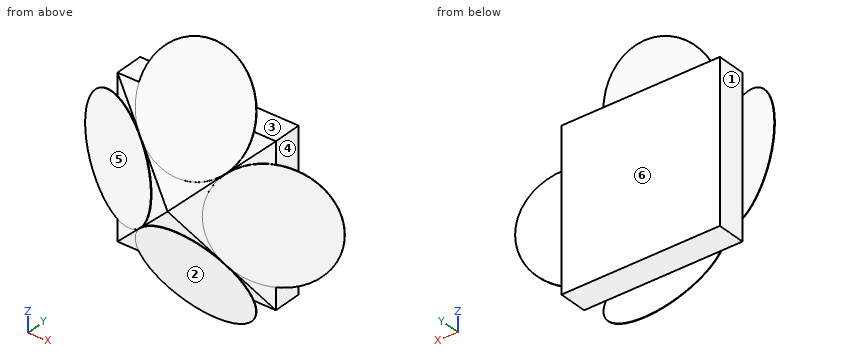
```python
from build123d import *

# Parameters (mm, degrees)
SALIENTE_EXTRUIR1_DEPTH = 32
CORTAR_EXTRUIR1_DEPTH   = 33
CROQUIS3_R              = 11.604472628
SALIENTE_EXTRUIR2_DEPTH = 0.1
CROQUIS4_R              = 11.609993134
SALIENTE_EXTRUIR3_DEPTH = 0.1
CROQUIS6_R              = 11.602426911
SALIENTE_EXTRUIR4_DEPTH = 0.1
CROQUIS7_R              = 11.59621687
SALIENTE_EXTRUIR5_DEPTH = 0.1


with BuildPart() as part:
    # Croquis1 → Saliente-Extruir1 (new body)
    with BuildSketch(Plane.XY):
        Polygon((-51.959662641, 8.927829358), (-51.959662641, 3.148169014), (-35.959662641, -4.290206314), (-19.959662641, 3.148169014), (-19.959662641, 8.927829358), align=None)
    extrude(amount=SALIENTE_EXTRUIR1_DEPTH)

    # Croquis2 → Cortar-Extruir1 (cut)
    with BuildSketch(Plane(origin=(-19.959662641, 0, 0), x_dir=(0, 0, -1), z_dir=(1, 0, 0))):
        Polygon((0, -4.290206314), (-16, -4.290206314), (0, 3.148169014), align=None)
        Polygon((-32, -4.290206314), (-32, 3.148169014), (-16, -4.290206314), align=None)
    extrude(amount=-CORTAR_EXTRUIR1_DEPTH, mode=Mode.SUBTRACT)

    # Croquis3 → Saliente-Extruir2 (add)
    with BuildSketch(Plane(origin=(-4.750700642, 10.218791996, 0), x_dir=(-0.9067966272160485, -0.42156835373353035, 0), z_dir=(0.42156835373353035, -0.9067966272160485, 0))):
        with Locations(Location((17.141516117, -16, 0), (0, 0, 312.201634939))):
            Circle(CROQUIS3_R)
    extrude(amount=SALIENTE_EXTRUIR2_DEPTH)

    # Croquis4 → Saliente-Extruir3 (add)
    with BuildSketch(Plane(origin=(0, -9.644179557, 4.483564205), x_dir=(-1, 0, 0), z_dir=(0, -0.9067966272160485, 0.4215683537335304))):
        with Locations(Location((35.959662641, -29.983548914, 0), (0, 0, 181.782387553))):
            Circle(CROQUIS4_R)
    extrude(amount=SALIENTE_EXTRUIR3_DEPTH)

    # Croquis6 → Saliente-Extruir4 (add)
    with BuildSketch(Plane(origin=(-8.030792992, -17.274294748, 0), x_dir=(-0.9067966272160486, 0.4215683537335302, 0), z_dir=(-0.4215683537335302, -0.9067966272160486, 0))):
        with Locations(Location((48.071640088, -16, 0), (0, 0, 271.839200589))):
            Circle(CROQUIS6_R)
    extrude(amount=SALIENTE_EXTRUIR4_DEPTH)

    # Croquis7 → Saliente-Extruir5 (add)
    with BuildSketch(Plane(origin=(0, 2.588676805, 1.203471855), x_dir=(-1, 0, 0), z_dir=(0, -0.9067966272160485, -0.4215683537335304))):
        with Locations(Location((35.959662641, 0.945548569, 0), (0, 0, 317.815283521))):
            Circle(CROQUIS7_R)
    extrude(amount=SALIENTE_EXTRUIR5_DEPTH)


solid = part.part
```
Read the model definition and answer for the solid it produces. Units are mm, in the model's axes. Face numbers are marked on the shaded views. A direction names the side the tool comes from. Coordinates: 2 decimals unless noted, no trailing zeros. Loops run counter-clockwise (first coordinate to the right, second up) from the corner with the lowest first, then second, coordinate; pieces in that order, holes last.
(1) The mould has two halves that part along X. Classify the marked faces 4, 5 and 6: released by +X, released by -X, zero draft, split by the parting line, or undercut.
Solution:
face 4: undercut
face 5: released by -X
face 6: zero draft
(2) Flat-ended cylindrical pins translate along their axes: pin 1 Ø3 at (x, y) = (-34, 7.5) entering from +Z; pin 2 Ø3 at (y, z) = (5, 31.5) entering from +X; pin 3 Ø1 at (x, y) = (-21.5, 2.5) entering from +Z. Find the tip coordinate at first contact, or state that the pin passes through.
Solution:
pin 1: stops at z = 42.23
pin 2: stops at x = -19.96
pin 3: stops at z = 31.68
(3) The part is cut by section B-B (y = 5.25). Count the separate pieces of the cut face and the enclosed holes in it, and give its area (3 significant figures).
Solution:
separate pieces: 5
enclosed holes: 0
area: 1,040 mm2
(4) The part is cut by section A-A (z = 12.5). Determine the outline of the cut face in (x, y), and give its area (3 significant figures).
Solution:
outline: (-61.7, 7.56) - (-41.63, -1.76) - (-41.59, -1.67) - (-39.46, -2.66) - (-32.46, -2.66) - (-30.33, -1.67) - (-30.29, -1.76) - (-10.22, 7.57) - (-10.26, 7.66) - (-19.96, 3.15) - (-19.96, 8.93) - (-51.96, 8.93) - (-51.96, 3.15) - (-61.65, 7.65) - close
area: 303 mm2
(5) A tool of negligible diameter and unlimited length cuts with its end or side. For the marked faces 1, 2 and 3, from which of +Z, -Z, +X, -X, +Y, -Y can it reach the whole face along a straight path? Write none if from no direction.
Solution:
face 1: +Z, -Z, +Y
face 2: -Z, +X, -X, -Y
face 3: +X, -X, +Y
(6) The part is cut by section C-C (z = 19). Determine the outline of the cut face in (x, y).
Solution:
outline: (-61.83, 7.63) - (-41.5, -1.82) - (-41.46, -1.73) - (-38.96, -2.9) - (-32.96, -2.9) - (-30.46, -1.73) - (-30.42, -1.82) - (-10.09, 7.63) - (-10.13, 7.72) - (-19.96, 3.15) - (-19.96, 8.93) - (-51.96, 8.93) - (-51.96, 3.15) - (-61.79, 7.72) - close
(7) Consider line 1 along X through (y, z) = (7.75, 18); line 2 along X through (y, z) = (5.5, 13); line 3 along Z through (x, y) = (-41.5, 5). Determine where each line is inside the solid, lowest interval first.
Solution:
line 1: x = -62.01 to -61.86, -51.96 to -19.96, -10.06 to -9.9
line 2: x = -57.26 to -57.02, -51.96 to -19.96, -14.9 to -14.66
line 3: z = -4.22 to -3.98, 0 to 32, 35.98 to 36.22
